from build123d import *

# Parameters (mm, degrees)
ESBO_O1_W                = 13.25
ESBO_O1_H                = 12.5
RESSALTO_EXTRUS_O1_DEPTH = 4.65
ESBO_O2_W                = 13.25
ESBO_O2_H                = 32.05
RESSALTO_EXTRUS_O2_DEPTH = 5
ESBO_O3_W                = 13.25
ESBO_O3_H                = 4.65
RESSALTO_EXTRUS_O3_DEPTH = 12.5
ESBO_O4_W                = 13.25
ESBO_O4_H                = 5
RESSALTO_EXTRUS_O4_DEPTH = 10
ESBO_O5_W                = 13.25
ESBO_O5_H                = 5
RESSALTO_EXTRUS_O5_DEPTH = 10
ESBO_O6_R                = 1.5
CORTE_EXTRUS_O1_DEPTH    = 10
ESBO_O7_R                = 1
CORTE_EXTRUS_O2_DEPTH    = 48.87512604
ESBO_O8_R                = 1
CORTE_EXTRUS_O3_DEPTH    = 48.87512604


with BuildPart() as part:
    # Esboço1 → Ressalto-extrusão1 (new body)
    with BuildSketch(Plane(origin=(0, 0, 0), x_dir=(1, 0, 0), z_dir=(0, 1, 0))):
        with Locations((-15.112918198, -12.411797698)):
            Rectangle(ESBO_O1_W, ESBO_O1_H)
    extrude(amount=-RESSALTO_EXTRUS_O1_DEPTH)

    # Esboço2 → Ressalto-extrusão2 (add)
    with BuildSketch(Plane(origin=(0, 0, 6.161797698), x_dir=(-1, 0, 0), z_dir=(0, 0, -1))):
        with Locations((15.112918198, -16.025)):
            Rectangle(ESBO_O2_W, ESBO_O2_H)
    extrude(amount=RESSALTO_EXTRUS_O2_DEPTH)

    # Esboço3 → Ressalto-extrusão3 (add)
    with BuildSketch(Plane.XY.offset(6.161797698)):
        with Locations((-15.112918198, -29.725)):
            Rectangle(ESBO_O3_W, ESBO_O3_H)
    extrude(amount=RESSALTO_EXTRUS_O3_DEPTH)

    # Esboço4 → Ressalto-extrusão4 (add)
    with BuildSketch(Plane(origin=(0, -32.05, 0), x_dir=(-1, 0, 0), z_dir=(0, -1, 0))):
        with Locations((15.112918198, -16.161797698)):
            Rectangle(ESBO_O4_W, ESBO_O4_H)
    extrude(amount=RESSALTO_EXTRUS_O4_DEPTH)

    # Esboço5 → Ressalto-extrusão5 (add)
    with BuildSketch(Plane(origin=(0, 0, 0), x_dir=(1, 0, 0), z_dir=(0, 1, 0))):
        with Locations((-15.112918198, -16.161797698)):
            Rectangle(ESBO_O5_W, ESBO_O5_H)
    extrude(amount=RESSALTO_EXTRUS_O5_DEPTH)

    # Esboço6 → Corte-extrusão1 (cut)
    with BuildSketch(Plane(origin=(0, 0, 13.661797698), x_dir=(-1, 0, 0), z_dir=(0, 0, -1))):
        with Locations((15.112918198, 5)):
            Circle(ESBO_O6_R)
        with Locations((15.112918198, -37.05)):
            Circle(ESBO_O6_R)
    extrude(amount=-CORTE_EXTRUS_O1_DEPTH, mode=Mode.SUBTRACT)

    # Esboço7 → Corte-extrusão2 (cut, through all)
    with BuildSketch(Plane(origin=(-8.487918198, 0, 0), x_dir=(0, 0, -1), z_dir=(1, 0, 0))):
        with Locations((-12.411797698, -2.325)):
            Circle(ESBO_O7_R)
    extrude(amount=-CORTE_EXTRUS_O2_DEPTH, mode=Mode.SUBTRACT)

    # Esboço8 → Corte-extrusão3 (cut, through all)
    with BuildSketch(Plane(origin=(-8.487918198, 0, 0), x_dir=(0, 0, -1), z_dir=(1, 0, 0))):
        with Locations((-12.411797698, -29.725)):
            Circle(ESBO_O8_R)
    extrude(amount=-CORTE_EXTRUS_O3_DEPTH, mode=Mode.SUBTRACT)


solid = part.part
The model under review builds one solid part; all positions refer to its coordinate system, in mm. A direction names the side the tool comes from. Round coordinates to 2 decimals unless told otherwise and drop trailing zeros. Loops run counter-clockwise (first coordinate to the right, second up) from the corner with the lowest first, then second, coordinate; pieces in that order, holes last. Notation, with made-up numbers: (39.25, -37.75) -> (76.25, -37.75) arc R21 ccw to (76.25, -21.75) -> close; hole circle Ø8 at (38.25, -1). An arc over 180 degrees is marked (long way). One line per question, with ' | ' between items. Start each with the question number.
Item 1: For pin 1 (3 mm diameter, centred on x = -17.5, y = 6, fed in from -Z); pin 2 (6 mm diameter, centred on x = -12.5, z = 5.5, fed in from -Y); pin 3 (4 mm diameter, centred on x = -18, z = 5.5, fed in from +Y); pin 4 (1.5 mm diameter, centred on y = -34, z = 4, fed in from -X), all flat-tipped, find the tip position at first contact; note any pin that passes through.
Item 2: Draft analysis for pull direction Z (two halves, no side actions). For faces 1 (the face through (-15.02, -2.02, 11.46)), 2 (the face through (-15, -27.4, 12)), 3 (the face through (-17, 5, 13.662)), 4 (the face through (-15.02, -28.734, 12.542)), state which applies: +Z half, -Z half, draft (parallel to the pull), parting line (faces both ways), or undercut.
Item 3: Add section B-B, the plane y = 5. Write out the cut boundary in (x, z).
Item 4: Wall thickness on line 1 along Y through (x, z) = (-11.5, 15.75); line 2 along Y through (x, z) = (-12.25, 10.5); line 3 along Y through (x, z) = (-14, 11.5): over which ranges is each line inside the solid? List them lowest first. Write a range as [from, to].
Item 5: Add section D-D, the plane z = 4.5. Write out the cut boundary in (x, y), then the cut area to 3 significant figures.
Item 6: Add section C-C, the plane z = 10.5. Write out the cut boundary in (x, y).
Item 7: Machinability: for faces 5 (the face through (-8.488, -16, 6)), 6 (the face through (-15, 0, 7)), 7 (the face through (-15, -32.05, 7)), 8 (the face through (-13.614, 5.066, 16.127)), 9 (the face through (-15, -4.65, 12)), which of the approach directions +Z, -Z, +X, -X, +Y, -Y give a long, thin tool a straight path to every point of the face, cutting with its end or side? Answer none if there is none.
Item 8: Add section A-A, the plane x = -16. Write out the cut boundary in (y, z) (3 decimals), then the cut area to 3 significant figures.
Return value:
1) pin 1: stops at z = 13.66 | pin 2: stops at y = -32.05 | pin 3: stops at y = 0 | pin 4: passes through
2) face 1: undercut | face 2: draft | face 3: -Z half | face 4: undercut
3) outline: (-21.74, 13.66) -> (-16.61, 13.66) -> (-16.61, 18.66) -> (-21.74, 18.66) -> close; (-13.61, 13.66) -> (-8.49, 13.66) -> (-8.49, 18.66) -> (-13.61, 18.66) -> close
4) line 1: y = [-42.05, -27.4], [-4.65, 10] | line 2: y = [-32.05, -27.4], [-4.65, 0] | line 3: y = [-32.05, -30.14], [-29.31, -27.4], [-4.65, -2.74], [-1.91, 0]
5) outline: (-21.74, -32.05) -> (-8.49, -32.05) -> (-8.49, 0) -> (-21.74, 0) -> close | area: 425 mm2
6) outline: (-21.74, -32.05) -> (-8.49, -32.05) -> (-8.49, -27.4) -> (-21.74, -27.4) -> close; (-21.74, -4.65) -> (-8.49, -4.65) -> (-8.49, 0) -> (-21.74, 0) -> close
7) face 5: +Z, -Z, +X, +Y, -Y | face 6: -Z, +X, -X, +Y | face 7: -Z, +X, -X, -Y | face 8: +Z, -Z | face 9: +Z, +X, -X
8) outline: (-42.05, 13.662) -> (-38.26, 13.662) -> (-38.26, 18.662) -> (-42.05, 18.662) -> close; (-35.84, 13.662) -> (-32.05, 13.662) -> (-32.05, 1.162) -> (0, 1.162) -> (0, 13.662) -> (3.79, 13.662) -> (3.79, 18.662) -> (-4.65, 18.662) -> (-4.65, 6.162) -> (-27.4, 6.162) -> (-27.4, 18.662) -> (-35.84, 18.662) -> close; (6.21, 13.662) -> (10, 13.662) -> (10, 18.662) -> (6.21, 18.662) -> close; hole circle Ø2 at (-29.725, 12.412); hole circle Ø2 at (-2.325, 12.412) | area: 346 mm2
